from build123d import *
from build123d.topology import SkipClean

# Parameters (mm, degrees)
BOSS_EXTRUDE1_DEPTH = 25
SKETCH2_R           = 8
CUT_EXTRUDE1_DEPTH  = 110
CUT_EXTRUDE2_DEPTH  = 150
BOSS_EXTRUDE2_START = 21.60254038
BOSS_EXTRUDE2_DEPTH = 21.60254038
SKETCH5_R           = 13
CUT_EXTRUDE3_DEPTH  = 50
SKETCH6_R           = 13
BOSS_EXTRUDE3_DEPTH = 100
SKETCH7_R           = 5
CUT_EXTRUDE4_DEPTH  = 50
SKETCH8_R           = 13
SKETCH8_R_2         = 5
BOSS_EXTRUDE4_DEPTH = 13
CUT_EXTRUDE5_DEPTH  = 28
SKETCH10_R          = 5
BOSS_EXTRUDE5_DEPTH = 10
CIRPATTERN2_COUNT   = 2
SKETCH11_W          = 47
SKETCH11_H          = 26
BOSS_EXTRUDE6_DEPTH = 10
SKETCH12_R          = 13
BOSS_EXTRUDE7_DEPTH = 67.86279097


with BuildPart() as part:
    # Sketch1 → Boss-Extrude1 (new, symmetric)
    with BuildSketch(Plane(origin=(0, 0, 0), x_dir=(1, 0, 0), z_dir=(0, 1, 0))):
        Polygon((86.602540378, 150), (103.923048454, 160), (114.724318643, 141.291651246), (93.073683549, 128.791651246), (158.073683549, 16.208348754), (179.724318643, 28.708348754), (190.525588833, 10), (173.205080757, 0), (45.59802172, 0), (22.79901086, 39.489045172), align=None)
    extrude(amount=BOSS_EXTRUDE1_DEPTH, both=True)

    # Sketch2 → Cut-Extrude1 (cut, symmetric)
    with BuildSketch(Plane(origin=(140.729128115, 0, -81.25), x_dir=(0.8660254037844386, 0, -0.5000000000000003), z_dir=(0.5000000000000003, 0, 0.8660254037844386))):
        Circle(SKETCH2_R)
    extrude(amount=CUT_EXTRUDE1_DEPTH, both=True, mode=Mode.SUBTRACT)

    # Sketch3 → Cut-Extrude2 (cut, symmetric)
    with BuildSketch(Plane(origin=(140.729128115, 0, -81.25), x_dir=(0.8660254037844386, 0, -0.5000000000000003), z_dir=(0.5000000000000003, 0, 0.8660254037844386))):
        with BuildLine():
            Line((0, 18), (-12.5, 18))
            Line((-12.5, 18), (-12.5, 31.312178452))
            Line((-12.5, 31.312178452), (23.905899442, 31.312178452))
            Line((23.905899442, 31.312178452), (23.905899442, -29.505210198))
            Line((23.905899442, -29.505210198), (-12.5, -29.505210198))
            Line((-12.5, -29.505210198), (-12.5, -18))
            Line((-12.5, -18), (0, -18))
            ThreePointArc((0, -18), (18, 0), (0, 18))
        make_face()
    extrude(amount=CUT_EXTRUDE2_DEPTH, both=True, mode=Mode.SUBTRACT)

    # Sketch4 → Boss-Extrude2 (add)
    with SkipClean():  # the faces are left unmerged after this step: merging them gives an invalid solid
        with BuildSketch(Plane(origin=(173.229128115, 0, -24.958348754), x_dir=(0.8660254037844386, 0, -0.5000000000000003), z_dir=(0.5000000000000003, 0, 0.8660254037844386)).offset(BOSS_EXTRUDE2_START)):
            with BuildLine():
                Line((7.5, 16.363068172), (7.5, 2.783882181))
                ThreePointArc((7.5, 2.783882181), (8, 0), (7.5, -2.783882181))
                Line((7.5, -2.783882181), (7.5, -16.363068172))
                ThreePointArc((7.5, -16.363068172), (18, 0), (7.5, 16.363068172))
            make_face()
        boss_extrude2 = extrude(amount=-BOSS_EXTRUDE2_DEPTH)

    # Mirror2: Boss-Extrude2 across plane
    with SkipClean():  # the faces are left unmerged after this step: merging them gives an invalid solid
        add(boss_extrude2.mirror(Plane(origin=(140.729128115, 0, -81.25), x_dir=(-0.8660254037844388, 0, 0.5), z_dir=(0.5000000000000003, 0, 0.8660254037844386))))

    # Sketch5 → Cut-Extrude3 (cut)
    with SkipClean():  # the faces are left unmerged after this step: merging them gives an invalid solid
        with BuildSketch(Plane(origin=(34.19851629, 0, -19.744522586), x_dir=(0.5000000000000001, 0, 0.8660254037844386), z_dir=(-0.8660254037844386, 0, 0.5000000000000001))):
            Circle(SKETCH5_R)
        extrude(amount=-CUT_EXTRUDE3_DEPTH, mode=Mode.SUBTRACT)


with BuildPart() as body_2:
    # Sketch6 → Boss-Extrude3 (new body)
    with BuildSketch(Plane(origin=(77.499786479, 0, -44.744522586), x_dir=(0.5000000000000001, 0, 0.8660254037844386), z_dir=(-0.8660254037844386, 0, 0.5000000000000001))):
        with Locations(Location((0, 0, 0), (0, 0, 180))):
            Circle(SKETCH6_R)
    extrude(amount=BOSS_EXTRUDE3_DEPTH)

    # Sketch7 → Cut-Extrude4 (cut, symmetric)
    with BuildSketch(Plane(origin=(140.729128115, 0, -81.25), x_dir=(0.8660254037844386, 0, -0.5000000000000003), z_dir=(0.5000000000000003, 0, 0.8660254037844386))):
        with Locations(Location((-162.5, 0, 0), (0, 0, 180.000000003))):
            Circle(SKETCH7_R)
    extrude(amount=CUT_EXTRUDE4_DEPTH, both=True, mode=Mode.SUBTRACT)

    # Sketch8 → Boss-Extrude4 (add, symmetric)
    with BuildSketch(Plane(origin=(140.729128115, 0, -81.25), x_dir=(0.8660254037844386, 0, -0.5000000000000003), z_dir=(0.5000000000000003, 0, 0.8660254037844386))):
        with Locations((-162.5, 0)):
            Circle(SKETCH8_R)
        with Locations((-162.5, 0)):
            Circle(SKETCH8_R_2, mode=Mode.SUBTRACT)
    extrude(amount=BOSS_EXTRUDE4_DEPTH, both=True)

    # Sketch9 → Cut-Extrude5 (cut, symmetric)
    with BuildSketch(Plane(origin=(140.729128115, 0, -81.25), x_dir=(0.8660254037844386, 0, -0.5000000000000003), z_dir=(0.5000000000000003, 0, 0.8660254037844386))):
        with BuildLine():
            Line((-162.5, 13), (-162.5, 18.834095503))
            ThreePointArc((-162.5, 18.834095503), (-181.334095503, 0), (-162.5, -18.834095503))
            Line((-162.5, -18.834095503), (-162.5, -13))
            ThreePointArc((-162.5, -13), (-175.5, 0), (-162.5, 13))
        make_face()
    extrude(amount=CUT_EXTRUDE5_DEPTH, both=True, mode=Mode.SUBTRACT)


with BuildPart() as body_2_2:
    # Sketch10 → Boss-Extrude5 (new body)
    with BuildSketch(Plane(origin=(6.75, 0, 11.691342951), x_dir=(0.8660254037844385, 0, -0.5000000000000004), z_dir=(0.5000000000000003, 0, 0.8660254037844384))):
        with BuildLine():
            Line((0, 13), (21.626254201, 13))
            Line((21.626254201, 13), (21.626254201, -13))
            Line((21.626254201, -13), (0, -13))
            ThreePointArc((0, -13), (-13, 0), (0, 13))
        make_face()
        Circle(SKETCH10_R, mode=Mode.SUBTRACT)
    extrude(amount=BOSS_EXTRUDE5_DEPTH)


with BuildPart() as cirpattern2_1:
    # CirPattern2: pattern copy
    add(body_2_2.part.rotate(Axis((0, 0, 0), (-0.8660254037844385, 0, 0.5000000000000003)), 1 * 360 / CIRPATTERN2_COUNT))


with BuildPart() as body_4:
    # Sketch11 → Boss-Extrude6 (new body)
    with BuildSketch(Plane(origin=(18.728885527, 0, -10.8131271), x_dir=(-0.5000000000000004, 0, -0.8660254037844385), z_dir=(0.8660254037844384, 0, -0.5000000000000003))):
        Rectangle(SKETCH11_W, SKETCH11_H)
    extrude(amount=-BOSS_EXTRUDE6_DEPTH)


with BuildPart() as body_5:
    # Sketch12 → Boss-Extrude7 (new body)
    with BuildSketch(Plane(origin=(18.728885527, 0, -10.8131271), x_dir=(-0.5000000000000004, 0, -0.8660254037844385), z_dir=(0.8660254037844384, 0, -0.5000000000000003))):
        with Locations(Location((0, 0, 0), (0, 0, 270))):
            Circle(SKETCH12_R)
    extrude(amount=BOSS_EXTRUDE7_DEPTH)


with BuildPart() as cirpattern2_1_1:
    add(cirpattern2_1.part)

    # Combine2: union body 4, body 5, body 2 2
    add(body_4.part)
    add(body_5.part)
    add(body_2_2.part)


solid = cirpattern2_1_1.part
Check sheet for the modelled part. Datum: model origin and axes. Units: mm. A direction names the side the tool comes from. Give positions to 0.01 mm unless a question says otherwise; leave off trailing zeros. Loops run counter-clockwise (first coordinate to the right, second up) from the corner with the lowest first, then second, coordinate; pieces in that order, holes last. Notation, with made-up numbers: M 57.5,69 L 67.5,69 A27 cw 67.5,105 Z; hole C 33.25,24 d10. An arc over 180 degrees is marked long. Return JSON: item names as keys, results as strings. Group by question number.
1. Thickness scan on L1, parallel to Y at x = 10.5, z = 18; L2, parallel to X at y = -2.75, z = -15; L3, parallel to X at y = 8, z = -24. Record the ranges inside material, lowest first.
2. Cross-section at A-A on y = 2.5. Record the boundary of the cut face in (x, z).
3. Mould release check, pull along X, two halves, no side actions. Record for faces 1 (the cylindrical face through (-20.47, 0.29, -9.46)), 2 (the flat face through (77.41, 0.18, -44.9)), 3 (the cylindrical face through (13.21, -1.92, 13.65)), 4 (the cylindrical face through (51.658, 10.316, -20.691)): released by +X, released by -X, zero draft, split by the parting line, or undercut.
4. Tool access check on faces 5 (the flat face through (11.044, -2.707, 9.212)), 6 (the flat face through (11, -13, -7)), 7 (the flat face through (10.163, 0.182, -5.649)). Record the directions out of +Z, -Z, +X, -X, +Y, -Y that give a thin tool (end or side, any length) a straight path to the whole face; none if there is none.
5. Cross-section at D-D on y = 11. Record the boundary of the cut face in (x, z), plus the area to 3 significant figures.
6. Go/stop test with flat-tipped pins: pin 1 (12 mm diameter, centred on x = 2.5, z = 17.5, fed in from -Y); pin 2 (4 mm diameter, centred on x = 59, y = -0.5, fed in from +Z); pin 3 (12 mm diameter, centred on x = 4, y = 0, fed in from -Z). Record where each tip stops, or that it passes through.
7. Cross-section at C-C on z = 3. Record the boundary of the cut face in (x, y).
8. Cross-section at B-B on y = -6.25. Record the boundary of the cut face in (x, z).
Return value:
{
 "1": {"L1": "-13 to -5, 5 to 13", "L2": "-21.02 to -13.48, -3.84 to -1.02, 4.76 to 51.39", "L3": "-5.43 to 11.12, 21.08 to 62.06"},
 "2": {"outline": "M -22.8,-13.97 L -15.5,-18.19 L -10.5,-9.53 L -17.8,-5.31 Z; M -8,-22.52 L 6.98,-31.16 L 12.35,-21.86 L 71.12,-55.79 L 83.88,-33.7 L 25.11,0.24 L 30.48,9.54 L 15.5,18.19 L 10.5,9.53 L 16.82,5.88 L 3.32,-17.5 L -3,-13.86 Z; M -4.3,18.07 L 3,13.86 L 8,22.52 L 0.7,26.73 Z"},
 "3": {"face 1": "released by -X", "face 2": "released by +X", "face 3": "undercut", "face 4": "undercut"},
 "4": {"face 5": "-X, +Y, -Y", "face 6": "+Z, -Z, +X, -X, -Y", "face 7": "+Y, -Y"},
 "5": {"outline": "M -17.75,-16.89 L 6.98,-31.16 L 15.26,-16.81 L 74.04,-50.74 L 80.96,-38.74 L 22.19,-4.81 L 30.48,9.54 L 5.75,23.82 L 0.75,15.16 L 16.82,5.88 L 3.32,-17.5 L -12.75,-8.23 Z", "area": "1,780 mm^2"},
 "6": {"pin 1": "y = -12.99", "pin 2": "z = -17.91", "pin 3": "z = -31.16"},
 "7": {"outline": "M 15.16,-13 L 26.7,-13 L 26.7,13 L 15.16,13 Z"},
 "8": {"outline": "M -21.62,-14.65 L 6.98,-31.16 L 13.03,-20.68 L 71.8,-54.62 L 83.2,-34.87 L 24.43,-0.94 L 30.48,9.54 L 1.88,26.05 L -3.12,17.39 L 16.82,5.88 L 3.32,-17.5 L -16.62,-5.99 Z"}
}
